```python
from build123d import *

# Parameters (mm, degrees)
SKETCH1_W            = 6
SKETCH1_H            = 6
EXTRUDE1_DEPTH       = 3.6
EXTRUDE2_DEPTH       = 0.35
MIRROR4_COPY_1_DEPTH = 0.35


with BuildPart() as part:
    # Sketch1 → Extrude1 (new body)
    with BuildSketch(Plane(origin=(0, 0, 0), x_dir=(1, 0, 0), z_dir=(0, 1, 0))):
        Rectangle(SKETCH1_W, SKETCH1_H)
    extrude(amount=EXTRUDE1_DEPTH)

    # Sketch2 → Revolve1 (revolve)
    with BuildSketch(Plane.XY.offset(2.25)):
        with BuildLine():
            Line((-2.25, 3.6), (-1.85, 3.6))
            ThreePointArc((-1.85, 3.6), (-1.967157288, 3.882842712), (-2.25, 4))
            Line((-2.25, 4), (-2.25, 3.6))
        make_face()
    revolve1 = revolve(axis=Axis((-2.25, 4.707394025, 2.25), (0, -1, 0)))

    # Mirror1: Revolve1 across plane
    add(revolve1.mirror(Plane.XY))

    # Mirror2: Revolve1 across plane
    add(revolve1.mirror(Plane(origin=(0, 0, 0), x_dir=(0, 0, 1), z_dir=(1, 0, 0))))

    # Mirror2 copy 1 sketch → Mirror2 copy 1 (revolve)
    with BuildSketch(Plane(origin=(0, 0, -2.25), x_dir=(-1, 0, 0), z_dir=(0, 0, -1))):
        with BuildLine():
            Line((-2.25, 3.6), (-1.85, 3.6))
            ThreePointArc((-1.85, 3.6), (-1.967157288, 3.882842712), (-2.25, 4))
            Line((-2.25, 4), (-2.25, 3.6))
        make_face()
    revolve(axis=Axis((2.25, 4.707394025, -2.25), (0, -1, 0)))

    # Sketch3 → Revolve2 (revolve)
    with BuildSketch(Plane.XY, mode=Mode.PRIVATE) as revolve2_sk:
        Polygon((-2.288507097, 3.6), (-1.75, 7), (0, 7), (0, 3.6), align=None)
    revolve(revolve2_sk.sketch.rotate(Axis((0, 7, 0), (0, -1, 0)), 270), axis=Axis((0, 7, 0), (0, -1, 0)))  # turned: the seam where the file's is

    # Sketch5 → Extrude2 (add, symmetric)
    with BuildSketch(Plane.XY.offset(2.25)):
        Polygon((-3, 1.05), (-3.25, 1.05), (-3.25, -0.25), (-2.215388365, -0.25), (-2.215388365, 0), (-3, 0), align=None)
    extrude2 = extrude(amount=EXTRUDE2_DEPTH, both=True)

    # Mirror3: Extrude2 across plane
    add(extrude2.mirror(Plane.XY))

    # Mirror4: Extrude2 across plane
    add(extrude2.mirror(Plane(origin=(0, 0, 0), x_dir=(0, 0, 1), z_dir=(1, 0, 0))))

    # Mirror4 copy 1 sketch → Mirror4 copy 1 (add, symmetric)
    with BuildSketch(Plane(origin=(0, 0, -2.25), x_dir=(-1, 0, 0), z_dir=(0, 0, -1))):
        Polygon((-3, 1.05), (-3.25, 1.05), (-3.25, -0.25), (-2.215388365, -0.25), (-2.215388365, 0), (-3, 0), align=None)
    extrude(amount=MIRROR4_COPY_1_DEPTH, both=True)


solid = part.part
```
Input: part model. Units: mm. Frame: model coordinates. Round coordinates to 2 decimals unless told otherwise and drop trailing zeros. Loops run counter-clockwise (first coordinate to the right, second up) from the corner with the lowest first, then second, coordinate; pieces in that order, holes last.
1) Section query B-B on z = 0. Return the cut outline in (x, y), plus the area to 3 significant figures.
Ans:
outline: (-3, 0) - (3, 0) - (3, 3.6) - (2.29, 3.6) - (1.75, 7) - (-1.75, 7) - (-2.29, 3.6) - (-3, 3.6) - close
area: 35.3 mm2
2) Section query D-D on x = 2.5. Return the cut outline in (y, z).
Ans:
outline: (-0.25, -2.6) - (0, -2.6) - (0, -3) - (3.6, -3) - (3.6, -2.56) arc R0.31 ccw to (3.6, -1.94) - (3.6, 1.94) arc R0.31 ccw to (3.6, 2.56) - (3.6, 3) - (0, 3) - (0, 2.6) - (-0.25, 2.6) - (-0.25, 1.9) - (0, 1.9) - (0, -1.9) - (-0.25, -1.9) - close
3) Pull-direction query (X, two-part tool) for faces 1 (the flat face through (0, 2, 3)), 2 (the flat face through (2, 3.6, -1.4)), 3 (the flat face through (0, 0, 0)); classes: released by +X, released by -X, zero draft, split by the parting line, or undercut.
Ans:
face 1: zero draft
face 2: undercut
face 3: undercut
4) Pin query (flat end, axial travel): pin 1 (3 mm diameter, centred on y = 1, z = 0.5, fed in from -X); pin 2 (1.5 mm diameter, centred on y = 3.5, z = 2, fed in from -X); pin 3 (1.5 mm diameter, centred on y = 2, z = 2, fed in from +X); pin 4 (1.5 mm diameter, centred on x = 0.5, z = 0, fed in from -Y). Return the tip coordinate at first contact, or that it passes through.
Ans:
pin 1: stops at x = -3.25
pin 2: stops at x = -3
pin 3: stops at x = 3
pin 4: stops at y = 0
5) Section query C-C on y = 0.75. Return the cut outline in (x, z), plus the area to 3 significant figures.
Ans:
outline: (-3.25, -2.6) - (-3, -2.6) - (-3, -3) - (3, -3) - (3, -2.6) - (3.25, -2.6) - (3.25, -1.9) - (3, -1.9) - (3, 1.9) - (3.25, 1.9) - (3.25, 2.6) - (3, 2.6) - (3, 3) - (-3, 3) - (-3, 2.6) - (-3.25, 2.6) - (-3.25, 1.9) - (-3, 1.9) - (-3, -1.9) - (-3.25, -1.9) - close
area: 36.7 mm2
6) Section query A-A on x = 0. Return the cut outline in (y, z), plus the area to 3 significant figures.
Ans:
outline: (0, -3) - (3.6, -3) - (3.6, -2.29) - (7, -1.75) - (7, 1.75) - (3.6, 2.29) - (3.6, 3) - (0, 3) - close
area: 35.3 mm2
7) Material intervals for line 1 (X direction, y = 2.5, z = 2.6); line 2 (Y direction, x = 2, z = 2.7); line 3 (Y direction, x = 1, z = -0.1), sorted ascending.
Ans:
line 1: x = -3 to 3
line 2: y = 0 to 3.6
line 3: y = 0 to 7
